Part model, mm, in its own coordinate system. A direction names the side the tool comes from. Give positions to 0.01 mm unless a question says otherwise; leave off trailing zeros. Order: outer loops, then holes, each group sorted by start corner. A loop starts at its lowest first (then second) coordinate and runs counter-clockwise, first axis right, second up. Notation, with made-up numbers: M 24.25,3.5 L 48.25,3.5 A24 ccw 48.25,28.5 Z; hole C 33.25,40.25 d1. An arc over 180 degrees is marked long. Write each question's results on one line, items separated by ' | '. Start each with the question number.
from build123d import *

# Parameters (mm, degrees)
SKETCH_1_R          = 29
EXTRUDE_1_DEPTH     = 6
SKETCH_2_R          = 3.1
CUT_EXTRUDE_1_DEPTH = 42.448763552
CUT_EXTRUDE_2_DEPTH = 42.448763552


with BuildPart() as part:
    # 草图1 → 凸台-拉伸1 (new body)
    with BuildSketch(Plane.XY):
        Circle(SKETCH_1_R)
    extrude(amount=EXTRUDE_1_DEPTH)

    # 草图2 → 切除-拉伸1 (cut, through all)
    with BuildSketch(Plane.XY.offset(6)):
        Circle(SKETCH_2_R)
    extrude(amount=-CUT_EXTRUDE_1_DEPTH, mode=Mode.SUBTRACT)

    # 草图3 → 切除-拉伸2 (cut, through all)
    with BuildSketch(Plane.XY.offset(6)):
        Polygon((-10, 10), (0, 20), (10, 10), align=None)
        Polygon((13.660254038, 3.660254038), (17.320508076, -10), (3.660254038, -13.660254038), align=None)
        Polygon((-3.660254038, -13.660254038), (-17.320508076, -10), (-13.660254038, 3.660254038), align=None)
    extrude(amount=-CUT_EXTRUDE_2_DEPTH, mode=Mode.SUBTRACT)


solid = part.part
(1) Pull direction Y, two halves, no side cores. Call faces 1 (the flat face through (5, 15, 3)), 2 (the cylindrical face through (13.38, -25.73, 2.96)), 3 (the flat face through (6, 0, 6)): +Y half, -Y half, draft (parallel to the pull), parting line (faces both ways), or undercut.
(2) Drop flat-ended pins along their axis: P1, Ø1.5, axis at y = 15, z = 1.5, coming from the +X side; P2, Ø6, axis at x = 15, y = -4.5, coming from the -Z side; P3, Ø3, axis at x = -2, z = 4.5, coming from the +Y side; P4, Ø3, axis at y = 23, z = 1.5, coming from the -X side. Give the stop position or say it passes through.
(3) Saw through at A-A on z = 3.75. Give the cut face in (x, y), plus the area to 3 significant figures.
(4) Saw through at C-C on y = 0. Give the cut face in (x, z).
(5) Saw through at B-B on x = -12. Give the cut face in (y, z), plus the area to 3 significant figures.
(6) Tool access for faces 4 (the flat face through (6, 0, 0)), 5 (the flat face through (-8.73, -4.88, 3.04)): list every direction of +Z, -Z, +X, -X, +Y, -Y with a clear straight run to the whole face (end or side of a thin tool).
(7) Probe L1, parallel to X at y = -6, z = 3; L2, parallel to Y at x = 1, z = 0.5; L3, parallel to X at y = -2.5, z = 1. List the from-to ranges inside material, lowest first.
(8) Saw through at D-D on y = 16. Give the cut face in (x, z), plus the area to 3 significant figures.
Taken from the geometry:
1) face 1: undercut | face 2: parting line | face 3: draft
2) P1: stops at x = 25.26 | P2: stops at z = 0 | P3: stops at y = 29 | P4: stops at x = -19.46
3) outline: C 0,0 d58; hole M -17.32,-10 L -3.66,-13.66 L -13.66,3.66 Z; hole M -10,10 L 10,10 L 0,20 Z; hole C 0,0 d6.2; hole M 3.66,-13.66 L 17.32,-10 L 13.66,3.66 Z | area: 2,310 mm²
4) outline: M -29,0 L -14.64,0 L -14.64,6 L -29,6 Z; M -11.55,0 L -3.1,0 L -3.1,6 L -11.55,6 Z; M 3.1,0 L 11.55,0 L 11.55,6 L 3.1,6 Z; M 14.64,0 L 29,0 L 29,6 L 14.64,6 Z
5) outline: M -26.4,0 L -11.43,0 L -11.43,6 L -26.4,6 Z; M 0.78,0 L 26.4,0 L 26.4,6 L 0.78,6 Z | area: 244 mm²
6) face 4: -Z, +X, -X, +Y, -Y | face 5: +Z, -Z
7) L1: x = -28.37 to -16.25, -8.08 to 8.08, 16.25 to 28.37 | L2: y = -28.98 to -2.93, 2.93 to 10, 19 to 28.98 | L3: x = -28.89 to -15.31, -10.1 to -1.83, 1.83 to 10.1, 15.31 to 28.89
8) outline: M -24.19,0 L -4,0 L -4,6 L -24.19,6 Z; M 4,0 L 24.19,0 L 24.19,6 L 4,6 Z | area: 242 mm²
